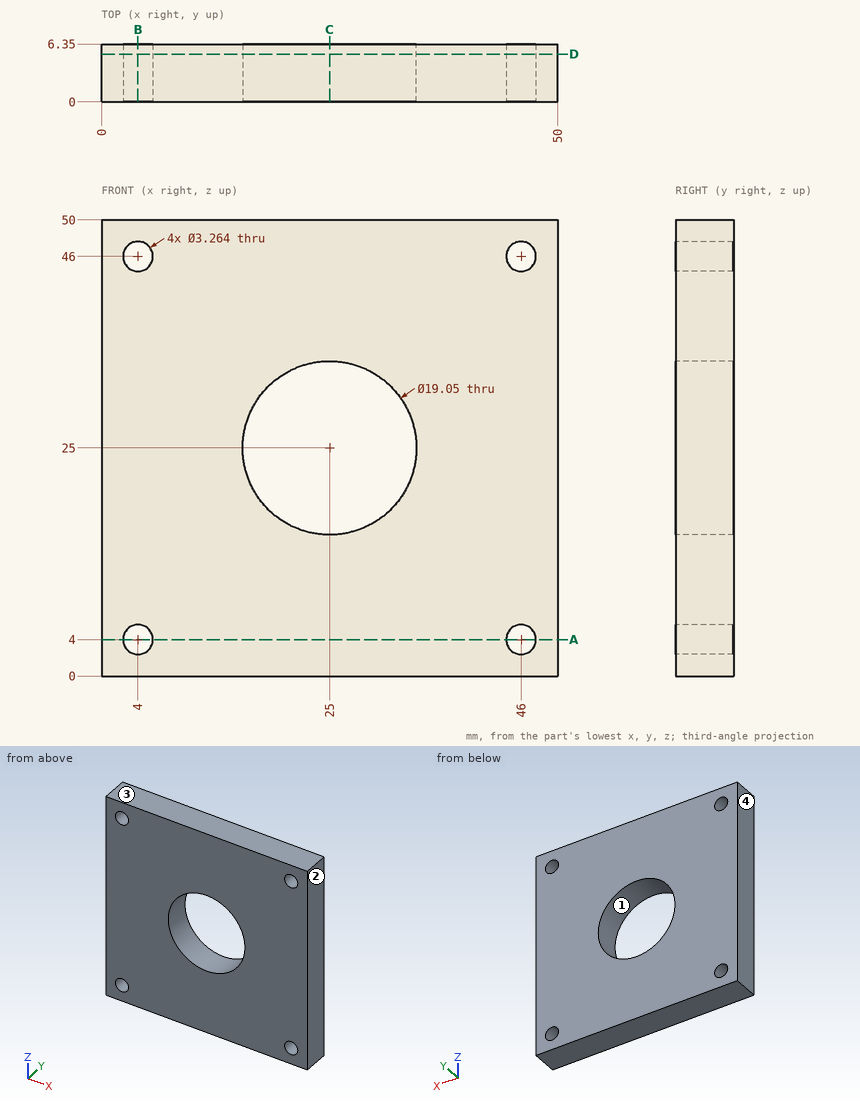
Answer from the drawing. Dimensions are ordinates in mm from the lowest x, y and z of the part. Coordinates: 2 decimals unless noted, no trailing zeros. Order: outer loops, then holes, each group sorted by start corner. A loop starts at its lowest first (then second) coordinate and runs counter-clockwise, first axis right, second up. Notation, with made-up numbers: (49, 86.5) -> (90, 86.5) arc R15 cw to (90, 110.5) -> close; hole circle Ø6 at (-21.75, -13). An arc over 180 degrees is marked (long way). Answer as a JSON object with one key per item and string values.
1) This flat-tipped pin is pushed along its axis until it touches: pin 1 (2.5 mm diameter, centred on x = 46, z = 4, fed in from +Y). Where does it stop, or does it pass through?
Model answer:
{"pin 1": "passes through"}
2) A cutting plane is placed at B-B, the plane x = 4. Determine the outline of the cut face in (y, z), plus the area to 3 significant figures.
Model answer:
{"outline": "(0, 0) -> (6.35, 0) -> (6.35, 2.37) -> (0, 2.37) -> close; (0, 5.63) -> (6.35, 5.63) -> (6.35, 44.37) -> (0, 44.37) -> close; (0, 47.63) -> (6.35, 47.63) -> (6.35, 50) -> (0, 50) -> close", "area": "276 mm²"}
3) A cutting plane is placed at A-A, the plane z = 4. Determine the outline of the cut face in (x, y).
Model answer:
{"outline": "(0, 0) -> (2.37, 0) -> (2.37, 6.35) -> (0, 6.35) -> close; (5.63, 0) -> (44.37, 0) -> (44.37, 6.35) -> (5.63, 6.35) -> close; (47.63, 0) -> (50, 0) -> (50, 6.35) -> (47.63, 6.35) -> close"}
4) A cutting plane is placed at C-C, the plane x = 25. Determine the outline of the cut face in (y, z) (3 decimals).
Model answer:
{"outline": "(0, 0) -> (6.35, 0) -> (6.35, 15.475) -> (0, 15.475) -> close; (0, 34.525) -> (6.35, 34.525) -> (6.35, 50) -> (0, 50) -> close"}
5) Consider line 1 along Z through (x, y) = (46, 2.5); line 2 along Z through (x, y) = (45, 0.75). Determine where each line is inside the solid, lowest interval first. Write a range as from..to.
Model answer:
{"line 1": "z = 0..2.37, 5.63..44.37, 47.63..50", "line 2": "z = 0..2.71, 5.29..44.71, 47.29..50"}
6) The mould has two halves that part along X. Classify the marked faces 1, 2, 3 and 4: released by +X, released by -X, zero draft, split by the parting line, or undercut.
Model answer:
{"face 1": "undercut", "face 2": "released by +X", "face 3": "zero draft", "face 4": "released by -X"}
7) A cutting plane is placed at D-D, the plane y = 5.25. Determine the outline of the cut face in (x, z) (3 decimals), plus the area to 3 significant figures.
Model answer:
{"outline": "(0, 0) -> (50, 0) -> (50, 50) -> (0, 50) -> close; hole circle Ø3.264 at (4, 4); hole circle Ø3.264 at (4, 46); hole circle Ø19.05 at (25, 25); hole circle Ø3.264 at (46, 4); hole circle Ø3.264 at (46, 46)", "area": "2,180 mm²"}
